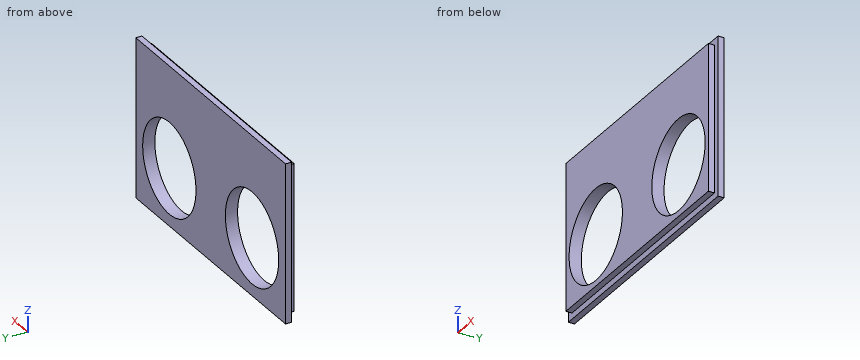
```python
from build123d import *

# Parameters (mm, degrees)
SKETCH1_W           = 105
SKETCH1_H           = 65
BOSS_EXTRUDE1_DEPTH = 5
SKETCH2_W           = 105
SKETCH2_H           = 65
SKETCH2_W_2         = 100
SKETCH2_H_2         = 60
CUT_EXTRUDE1_DEPTH  = 2.5
SKETCH3_R           = 18.7
CUT_EXTRUDE2_DEPTH  = 50


with BuildPart() as part:
    # Sketch1 → Boss-Extrude1 (new body)
    with BuildSketch(Plane(origin=(0, 0, 0), x_dir=(1, 0, 0), z_dir=(0, 1, 0))):
        Rectangle(SKETCH1_W, SKETCH1_H)
    extrude(amount=BOSS_EXTRUDE1_DEPTH)

    # Sketch2 → Cut-Extrude1 (cut)
    with BuildSketch(Plane.XZ):
        Rectangle(SKETCH2_W, SKETCH2_H)
        Rectangle(SKETCH2_W_2, SKETCH2_H_2, mode=Mode.SUBTRACT)
    extrude(amount=-CUT_EXTRUDE1_DEPTH, mode=Mode.SUBTRACT)

    # Sketch3 → Cut-Extrude2 (cut)
    with BuildSketch(Plane(origin=(0, 5, 0), x_dir=(1, 0, 0), z_dir=(0, 1, 0))):
        with Locations((-29, 9)):
            Circle(SKETCH3_R)
        with Locations((29, 9)):
            Circle(SKETCH3_R)
    extrude(amount=-CUT_EXTRUDE2_DEPTH, mode=Mode.SUBTRACT)


solid = part.part
```
Design review of the part built by this model. Coordinates are the model's own, in mm. Coordinates: 2 decimals unless noted, no trailing zeros. Write each loop counter-clockwise with the first axis right and the second up, starting at its lowest first coordinate (ties: lowest second). Pieces come first, ordered by that corner, then holes. Notation, with made-up numbers: M 76,-20.75 L 127,-20.75 A15 cw 127,-5.75 Z; hole C -3.75,83 d4. An arc over 180 degrees is marked long. Answer as a JSON object with one key per item and string values.
Item 1: Add section A-A, the plane x = 29. Give the boundary of the cut face in (y, z).
Outcome:
{"outline": "M 0,-30 L 2.5,-30 L 2.5,-32.5 L 5,-32.5 L 5,-27.7 L 0,-27.7 Z; M 0,9.7 L 5,9.7 L 5,32.5 L 2.5,32.5 L 2.5,30 L 0,30 Z"}
Item 2: Add section C-C, the plane y = 4.1. Give the boundary of the cut face in (x, z).
Outcome:
{"outline": "M -52.5,-32.5 L 52.5,-32.5 L 52.5,32.5 L -52.5,32.5 Z; hole C -29,-9 d37.4; hole C 29,-9 d37.4"}
Item 3: Wall thickness on probe 1 along X at (y, z) = (1.2, -9); probe 2 along X at (y, z) = (3, -9); probe 3 along Z at (x, y) = (-29, 2): over which ranges is each line inside the solid? List them lowest first.
Outcome:
{"probe 1": "-50 to -47.7, -10.3 to 10.3, 47.7 to 50", "probe 2": "-52.5 to -47.7, -10.3 to 10.3, 47.7 to 52.5", "probe 3": "-30 to -27.7, 9.7 to 30"}
Item 4: Add section D-D, the plane z = 19.5. Give the boundary of the cut face in (x, y).
Outcome:
{"outline": "M -52.5,2.5 L -50,2.5 L -50,0 L 50,0 L 50,2.5 L 52.5,2.5 L 52.5,5 L -52.5,5 Z"}
Item 5: Add section B-B, the plane z = -9. Give the boundary of the cut face in (x, y).
Outcome:
{"outline": "M -52.5,2.5 L -50,2.5 L -50,0 L -47.7,0 L -47.7,5 L -52.5,5 Z; M -10.3,0 L 10.3,0 L 10.3,5 L -10.3,5 Z; M 47.7,0 L 50,0 L 50,2.5 L 52.5,2.5 L 52.5,5 L 47.7,5 Z"}
Item 6: Insertion check: pin 1 Ø1.2 at (x, y) = (0.5, 2) entering from -Z; pin 2 Ø1.2 at (y, z) = (1, 0) entering from -X; pin 3 Ø1.2 at (x, y) = (-12, 1) entering from +Z; pin 4 Ø0.8 at (y, z) = (1.5, 3.5) entering from +X. Each pin has a flat end and moves straight along its axis. Give the tip position at first contact, or say it passes through.
Outcome:
{"pin 1": "z = -32.5", "pin 2": "x = -50", "pin 3": "z = 30", "pin 4": "x = 50"}
